Can you work these out from the model? Positions are in its coordinate system, mm. Round coordinates to 2 decimals unless told otherwise and drop trailing zeros. Order: outer loops, then holes, each group sorted by start corner. A loop starts at its lowest first (then second) coordinate and runs counter-clockwise, first axis right, second up. Notation, with made-up numbers: M -18.5,0 L -5.5,0 A24 ccw -5.5,13 Z; hole C 26.5,22 d10. An arc over 180 degrees is marked long. Answer as CSV lines item,"result". Start each with the question number.
from build123d import *

# Parameters (mm, degrees)
SKETCH1_R           = 1.5
SKETCH1_W           = 123.128854939
SKETCH1_H           = 42.830428858
BOSS_EXTRUDE1_DEPTH = 0.4


with BuildPart() as part:
    # Sketch1 → Boss-Extrude1 (new body)
    with BuildSketch(Plane.XY):
        with BuildLine():
            Line((1, 0), (139, 0))
            ThreePointArc((139, 0), (139.707106781, 0.292893219), (140, 1))
            Line((140, 1), (140, 55))
            ThreePointArc((140, 55), (139.707106781, 55.707106781), (139, 56))
            Line((139, 56), (1, 56))
            ThreePointArc((1, 56), (0.292893219, 55.707106781), (0, 55))
            Line((0, 55), (0, 1))
            ThreePointArc((0, 1), (0.292893219, 0.292893219), (1, 0))
        make_face()
        with Locations((5, 51.5)):
            Circle(SKETCH1_R, mode=Mode.SUBTRACT)
        with Locations((5, 4.5)):
            Circle(SKETCH1_R, mode=Mode.SUBTRACT)
        with Locations((135, 4.5)):
            Circle(SKETCH1_R, mode=Mode.SUBTRACT)
        with Locations((135, 51.5)):
            Circle(SKETCH1_R, mode=Mode.SUBTRACT)
        with Locations((70.169366708, 28.217965612)):
            Rectangle(SKETCH1_W, SKETCH1_H, mode=Mode.SUBTRACT)
    extrude(amount=-BOSS_EXTRUDE1_DEPTH)


solid = part.part
(1) I want a section at A-A on y = 51.5. Write out the boundary of the cut face in (x, z).
(2) I want a section at B-B on y = 31. Write out the boundary of the cut face in (x, z).
(3) If we mould it in two halves opening along Y, with no side actions, what happens to faces 1 (the cylindrical face through (4.675, 50.036, -0.197)), 2 (the flat face through (70, 51, 0))? For each: +Y half, -Y half, draft (parallel to the pull), parting line (faces both ways), or undercut.
(4) I want a section at D-D on x = 22.5. Write out the boundary of the cut face in (y, z).
(5) If I drill on line 1 along Y through (x, z) = (5, -0.05); line 2 along X through (y, z) = (23.5, -0.35); line 3 along Y through (x, z) = (67, -0.35), over which ranges is the centre line in solid material (lowest first)?
(6) I want a section at C-C on z = -0.1. Write out the boundary of the cut face in (x, y).
From the geometry:
1,outline,"M 0,-0.4 L 3.5,-0.4 L 3.5,0 L 0,0 Z; M 6.5,-0.4 L 133.5,-0.4 L 133.5,0 L 6.5,0 Z; M 136.5,-0.4 L 140,-0.4 L 140,0 L 136.5,0 Z"
2,outline,"M 0,-0.4 L 8.6,-0.4 L 8.6,0 L 0,0 Z; M 131.73,-0.4 L 140,-0.4 L 140,0 L 131.73,0 Z"
3,face 1,"undercut"
3,face 2,"draft"
4,outline,"M 0,-0.4 L 6.8,-0.4 L 6.8,0 L 0,0 Z; M 49.63,-0.4 L 56,-0.4 L 56,0 L 49.63,0 Z"
5,line 1,"0 to 3, 6 to 50, 53 to 56"
5,line 2,"0 to 8.6, 131.73 to 140"
5,line 3,"0 to 6.8, 49.63 to 56"
6,outline,"M 0,1 A1 ccw 1,0 L 139,0 A1 ccw 140,1 L 140,55 A1 ccw 139,56 L 1,56 A1 ccw 0,55 Z; hole C 5,4.5 d3; hole C 5,51.5 d3; hole M 8.6,6.8 L 131.73,6.8 L 131.73,49.63 L 8.6,49.63 Z; hole C 135,4.5 d3; hole C 135,51.5 d3"
